Could you check a few things on this model? Use its own coordinates, in mm. A direction names the side the tool comes from. Coordinates: 2 decimals unless noted, no trailing zeros. Loops run counter-clockwise (first coordinate to the right, second up) from the corner with the lowest first, then second, coordinate; pieces in that order, holes last.
from build123d import *

# Parameters (mm, degrees)
F0_R     = 2.794
F1_DEPTH = 4.826


with BuildPart() as f1:
    # F0 (on Front) → F1 (new body)
    with BuildSketch(Plane.XZ):
        with BuildLine():
            Line((-6.199785, -15.992633), (6.499093, -16.161406))
            Line((6.499093, -16.161406), (6.199785, -11.344696))
            ThreePointArc((6.199785, -11.344696), (12.927958, -0.085905), (6.35, 11.261304))
            Line((6.35, 11.261304), (6.35, 16.087304))
            Line((6.35, 16.087304), (-6.35, 16.087304))
            Line((-6.35, 16.087304), (-6.35, 11.261304))
            ThreePointArc((-6.35, 11.261304), (-12.927958, 0.085905), (-6.499093, -11.175923))
            Line((-6.499093, -11.175923), (-6.199785, -15.992633))
        make_face()
        Circle(F0_R, mode=Mode.SUBTRACT)
    extrude(amount=F1_DEPTH)


solid = f1.part
(1) Which directions (+Z, -Z, +X, -X, +Y, -Y) give clear straight access to the entire face, cutting with the end or side of a thin tool? Please do faces 4 (the face through (-2.217, -2.379, -1.7)), 5 (the face through (6.35, -2, 14)), 6 (the face through (-6.35, -2, 14)).
Answers:
face 4: +Y, -Y
face 5: +Z, +X, +Y, -Y
face 6: +Z, -X, +Y, -Y
(2) We'd pull the mould along Z, two halves only. Please class faces 1 (the face through (6.35, -2.38, -13.79)), 2 (the face through (-6.35, -2.38, -13.55)), 3 (the face through (-3, 0, 0)): +Z half, -Z half, draft (parallel to the pull), parting line (faces both ways), or undercut.
Answers:
face 1: undercut
face 2: -Z half
face 3: draft
(3) I need wall thicknesses on probe 1 along Z at (x, y) = (-6, -4.45); probe 2 along Z at (x, y) = (0, -3.15); probe 3 along X at (y, z) = (-3.8, -2.5). Which ranges of each line are inside material? Lowest first, please.
Answers:
probe 1: z = -16 to 16.09
probe 2: z = -16.08 to -2.79, 2.79 to 16.09
probe 3: x = -12.68 to -1.25, 1.25 to 12.68
(4) For pin 1 (1.4 mm diameter, centred on y = -1, z = 13, fed in from +X); pin 2 (1.5 mm diameter, centred on y = -2.5, z = 7, fed in from -X); pin 3 (1 mm diameter, centred on x = 2, y = -1.5, fed in from -Z), each with a flat end and sliding along its axis, tell me the tip position at first contact or that it passes through.
Answers:
pin 1: stops at x = 6.35
pin 2: stops at x = -11.32
pin 3: stops at z = -16.11
(5) Imagine slicing it at C-C, the plane x = 0. Write out the boundary of the cut face in (y, z), and give its area (3 significant figures).
Answers:
outline: (-4.83, -16.08) - (0, -16.08) - (0, -2.79) - (-4.83, -2.79) - close; (-4.83, 2.79) - (0, 2.79) - (0, 16.09) - (-4.83, 16.09) - close
area: 128 mm2
(6) Imagine slicing it at A-A, the plane z = 0. Write out the boundary of the cut face in (x, y).
Answers:
outline: (-12.93, -4.83) - (-2.79, -4.83) - (-2.79, 0) - (-12.93, 0) - close; (2.79, -4.83) - (12.93, -4.83) - (12.93, 0) - (2.79, 0) - close
(7) Imagine slicing it at B-B, the plane y = -1.7. Write out the boundary of the cut face in (x, z).
Answers:
outline: (-6.5, -11.18) - (-6.2, -15.99) - (6.5, -16.16) - (6.2, -11.34) arc R12.93 ccw to (6.35, 11.26) - (6.35, 16.09) - (-6.35, 16.09) - (-6.35, 11.26) arc R12.93 ccw to start; hole circle Ø5.59 at (0, 0)
(8) Imagine slicing it at D-D, the plane z = -7. Write out the boundary of the cut face in (x, y).
Answers:
outline: (-10.87, -4.83) - (10.87, -4.83) - (10.87, 0) - (-10.87, 0) - close
